Source: three-view drawing plus pictorial views. Frame: mm from the lowest corner of the part. Give positions to 0.01 mm unless a question says otherwise; leave off trailing zeros. Write each loop counter-clockwise with the first axis right and the second up, starting at its lowest first coordinate (ties: lowest second). Pieces come first, ordered by that corner, then holes. Notation, with made-up numbers: M 26,79.5 L 65,79.5 A21 cw 65,92.5 Z; hole C -15.75,28.25 d3. An arc over 180 degrees is marked long. Return JSON: item names as keys, results as strings.
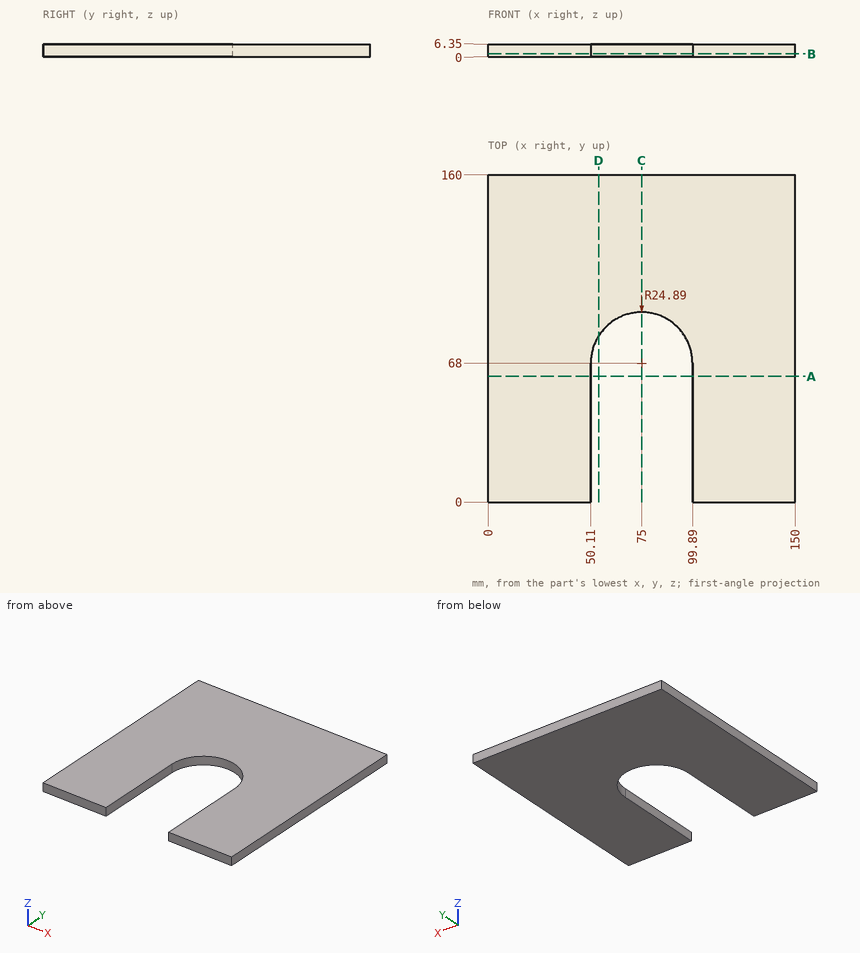
1) Cut plane D-D, the plane x = 54. Return the cut outline in (y, z).
Numbers:
{"outline": "M 81.36,0 L 160,0 L 160,6.35 L 81.36,6.35 Z"}
2) Cut plane A-A, the plane y = 61.5. Return the cut outline in (x, z), then the cut area to 3 significant figures.
Numbers:
{"outline": "M 0,0 L 50.11,0 L 50.11,6.35 L 0,6.35 Z; M 99.89,0 L 150,0 L 150,6.35 L 99.89,6.35 Z", "area": "636 mm²"}
3) Line query: line 1 (X direction, y = 8, z = 3.75); line 2 (Y direction, x = 82.5, z = 5); line 3 (Y direction, x = 52, z = 5.5). Output: solid intervals per line, ascending. Write a range as [from, to].
Numbers:
{"line 1": "x = [0, 50.11], [99.89, 150]", "line 2": "y = [91.73, 160]", "line 3": "y = [77.51, 160]"}
4) Cut plane B-B, the plane z = 1.5. Return the cut outline in (x, y), then the cut area to 3 significant figures.
Numbers:
{"outline": "M 0,0 L 50.11,0 L 50.11,68 A24.89 cw 99.89,68 L 99.89,0 L 150,0 L 150,160 L 0,160 Z", "area": "19,600 mm²"}
5) Cut plane C-C, the plane x = 75. Return the cut outline in (y, z).
Numbers:
{"outline": "M 92.89,0 L 160,0 L 160,6.35 L 92.89,6.35 Z"}
